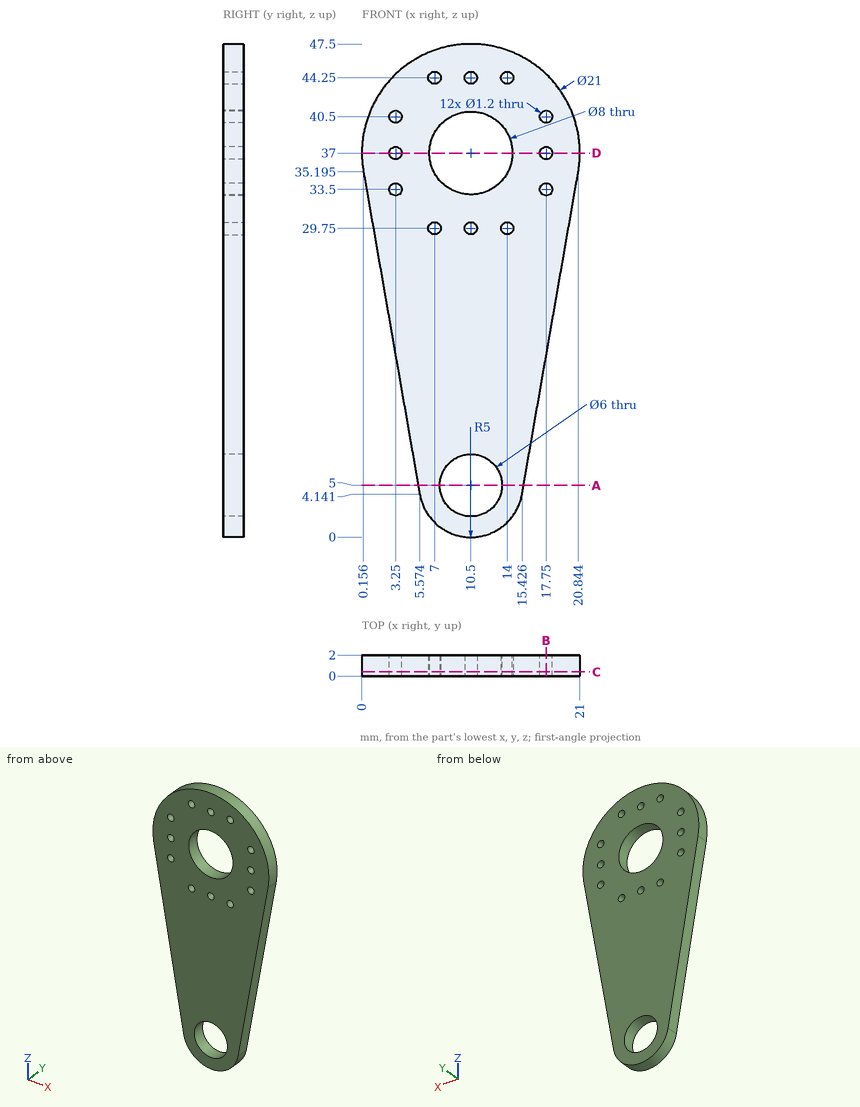
Answer from the drawing. Dimensions are ordinates in mm from the lowest x, y and z of the part. Coordinates: 2 decimals unless noted, no trailing zeros. Write each loop counter-clockwise with the first axis right and the second up, starting at its lowest first coordinate (ties: lowest second). Pieces come first, ordered by that corner, then holes. Notation, with made-up numbers: (-38, -34.75) - (-18, -34.75) arc R21 ccw to (-18, -9.75) - close; hole circle Ø9 at (20, -23.5). An arc over 180 degrees is marked (long way). One line per question, with ' | ' between items.
Q1. Find section C-C, the plane y = 0.4. State how many separate pieces and enclosed holes the cut face has, plus the area to 3 significant figures.
Result set:
separate pieces: 1 | enclosed holes: 14 | area: 624 mm^2
Q2. Consider L1, parallel to X at y = 0.45, z = 37; L2, parallel to X at y = 0.75, z = 44.25 (1 decimal); L3, parallel to Z at x = 10.25, y = 0.95 (1 decimal). Determine where each line is inside the solid, lowest interval first. Write a range as [from, to].
Result set:
L1: [0, 2.65], [3.85, 6.5], [14.5, 17.15], [18.35, 21] | L2: [2.9, 6.4], [7.6, 9.9], [11.1, 13.4], [14.6, 18.1] | L3: [0, 2], [8, 29.2], [30.3, 33], [41, 43.7], [44.8, 47.5]
Q3. Find section B-B, the plane x = 17.75. Write down the section's boundary in (y, z) (1 decimal).
Result set:
outline: (0, 17.5) - (2, 17.5) - (2, 32.9) - (0, 32.9) - close; (0, 34.1) - (2, 34.1) - (2, 36.4) - (0, 36.4) - close; (0, 37.6) - (2, 37.6) - (2, 39.9) - (0, 39.9) - close; (0, 41.1) - (2, 41.1) - (2, 44.6) - (0, 44.6) - close
Q4. This flat-tipped pin is pushed along its axis until it touches: P1, Ø1, axis at x = 10.5, z = 29.75, coming from the +Y side. Where does it stop, or does it pass through?
Result set:
P1: through
Q5. Find section A-A, the plane z = 5. Write down the section's boundary in (x, y) (1 decimal).
Result set:
outline: (5.4, 0) - (7.5, 0) - (7.5, 2) - (5.4, 2) - close; (13.5, 0) - (15.6, 0) - (15.6, 2) - (13.5, 2) - close
Q6. Find section D-D, the plane z = 37. Write down the section's boundary in (x, y).
Result set:
outline: (0, 0) - (2.65, 0) - (2.65, 2) - (0, 2) - close; (3.85, 0) - (6.5, 0) - (6.5, 2) - (3.85, 2) - close; (14.5, 0) - (17.15, 0) - (17.15, 2) - (14.5, 2) - close; (18.35, 0) - (21, 0) - (21, 2) - (18.35, 2) - close
